Read the model definition and answer for the solid it produces. Units are mm, in the model's axes. Round coordinates to 2 decimals unless told otherwise and drop trailing zeros. Write each loop counter-clockwise with the first axis right and the second up, starting at its lowest first coordinate (ties: lowest second). Pieces come first, ordered by that corner, then holes.
from build123d import *

# Parameters (mm, degrees)
SKETCH1_R               = 13.35
SKETCH1_R_2             = 11.24
BOSS_EXTRUDE1_DEPTH     = 1100
CUT_EXTRUDE1_DEPTH      = 1101.162008524
CUT_EXTRUDE1_DEPTH_BACK = 1101.162008524
SKETCH2_R               = 50
CUT_EXTRUDE2_DEPTH      = 1101.162008627
CUT_EXTRUDE2_DEPTH_BACK = 1101.162008627
SKETCH3_R               = 2231.362480005
SKETCH3_R_2             = 1050


with BuildPart() as part:
    # Sketch1 → Boss-Extrude1 (new body)
    with BuildSketch(Plane.XY):
        Circle(SKETCH1_R)
        Circle(SKETCH1_R_2, mode=Mode.SUBTRACT)
    extrude(amount=BOSS_EXTRUDE1_DEPTH)

    # Sketch2 → Cut-Extrude1 (cut, two sides: drawn at the far end of the back side and taken through both)
    with BuildSketch(Plane(origin=(0, 0, 0), x_dir=(0, 0, -1), z_dir=(1, 0, 0)).offset(-CUT_EXTRUDE1_DEPTH_BACK)):
        Circle(SKETCH2_R)
    extrude(amount=CUT_EXTRUDE1_DEPTH + CUT_EXTRUDE1_DEPTH_BACK, mode=Mode.SUBTRACT)

    # Sketch3 → Cut-Extrude2 (cut, two sides: drawn at the far end of the back side and taken through both)
    with BuildSketch(Plane(origin=(0, 0, 0), x_dir=(0, 0, -1), z_dir=(1, 0, 0)).offset(-CUT_EXTRUDE2_DEPTH_BACK)):
        Circle(SKETCH3_R)
        Circle(SKETCH3_R_2, mode=Mode.SUBTRACT)
    extrude(amount=CUT_EXTRUDE2_DEPTH + CUT_EXTRUDE2_DEPTH_BACK, mode=Mode.SUBTRACT)


solid = part.part
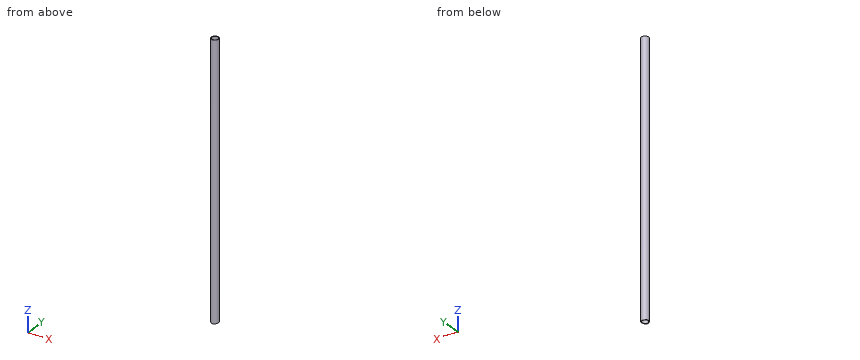
Q1. Section B-B (x = -2.75) is taken. Determine the outline of the cut face in (y, z), then the cut area to 3 significant figures.
Verdict:
outline: (-13.06, 48.26) arc R50 cw to (-10.9, 48.8) - (-10.9, 1049.94) arc R1050 ccw to (-13.06, 1049.92) - close; (10.9, 48.8) arc R50 cw to (13.06, 48.26) - (13.06, 1049.92) arc R1050 ccw to (10.9, 1049.94) - close
area: 4,340 mm2
Q2. Flat-ended cylindrical pins translate along their axes: pin 1 Ø3 at (y, z) = (6.5, 334.5) entering from -X; pin 2 Ø2 at (y, z) = (-1.5, 161) entering from -X; pin 3 Ø1 at (x, z) = (4.5, 445) entering from +Y. Find the tip coordinate at first contact, or state that the pin passes through.
Verdict:
pin 1: stops at x = -12.38
pin 2: stops at x = -13.34
pin 3: stops at y = 12.74
Q3. Section A-A (y = 0) is taken. Determine the outline of the cut face in (x, z), then the cut area to 3 significant figures.
Verdict:
outline: (-13.35, 50) - (-11.24, 50) - (-11.24, 1050) - (-13.35, 1050) - close; (11.24, 50) - (13.35, 50) - (13.35, 1050) - (11.24, 1050) - close
area: 4,220 mm2
Q4. Section C-C (z = 891) is taken. Determine the outline of the cut face in (x, y).
Verdict:
outline: circle Ø26.7 at (0, 0); hole circle Ø22.48 at (0, 0)
Q5. Straight lines are drawn through the part: probe 1 along X at (y, z) = (0, 270); probe 2 along Y at (x, z) = (-1, 875.5); probe 3 along Z at (x, y) = (-6.5, 10.75). For each, find the intervals that lie inside material, in ascending order.
Verdict:
probe 1: x = -13.35 to -11.24, 11.24 to 13.35
probe 2: y = -13.31 to -11.2, 11.2 to 13.31
probe 3: z = 48.83 to 1049.94
